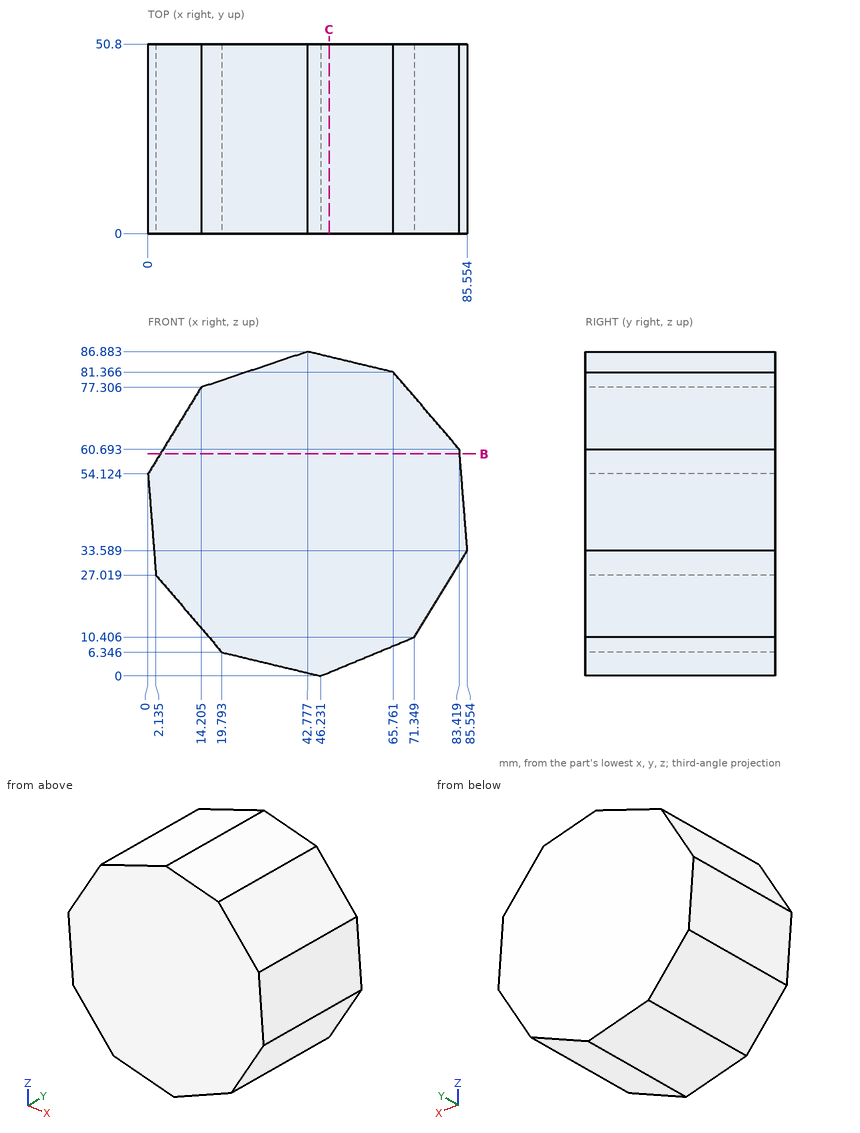
Design review of the part shown in the three views and the two pictorial views. Dimensions are in mm from the part's minimum x, y and z. Give positions to 0.01 mm unless a question says otherwise; leave off trailing zeros. Write each loop counter-clockwise with the first axis right and the second up, starting at its lowest first coordinate (ties: lowest second). Pieces come first, ordered by that corner, then holes. Notation, with made-up numbers: M -0.5,-0.5 L 9.5,-0.5 A13 cw 9.5,23.5 Z; hole C -16,-6.75 d4. An arc over 180 degrees is marked long. Return JSON: item names as keys, results as strings. Group by question number.
Item 1: Take a section at B-B (z = 59.5). Give the boundary of the cut face in (x, y) (1 decimal).
Item 2: Clearance check with flat-ended pins moving along their axes: pin 1 Ø6 at (x, y) = (60.5, 29.5) entering from +Z; pin 2 Ø1 at (x, y) = (75.5, 22) entering from -Z (1 decimal); pin 3 Ø12 at (x, y) = (64.5, 25.5) entering from +Z. State where each tip first meets the part, or that it passes through.
Item 3: Wall thickness on line 1 along Z through (x, y) = (71, 25) (1 decimal); line 2 along X through (y, z) = (38, 67); line 3 along X through (y, z) = (14.5, 33.5) (1 decimal): over which ranges is each line inside the solid? List them lowest first.
Item 4: Take a section at C-C (x = 48.5). Give the boundary of the cut face in (y, z), plus the area to 3 significant figures.
Return value:
{
 "1": {"outline": "M 3.3,0 L 83.5,0 L 83.5,50.8 L 3.3,50.8 Z"},
 "2": {"pin 1": "stops at z = 83.35", "pin 2": "stops at z = 16.4", "pin 3": "stops at z = 83.11"},
 "3": {"line 1": "z = 10.3 to 75.2", "line 2": "x = 7.89 to 78.03", "line 3": "x = 1.6 to 85.5"},
 "4": {"outline": "M 0,0.94 L 50.8,0.94 L 50.8,85.51 L 0,85.51 Z", "area": "4,300 mm2"}
}
